Source: CAD feature listing. Evaluate the final solid. Frame: model axes, mm. Face numbers are marked on the shaded views. A direction names the side the tool comes from. Give positions to 0.01 mm unless a question says otherwise; leave off trailing zeros. Write each loop counter-clockwise with the first axis right and the second up, starting at its lowest first coordinate (ties: lowest second). Pieces come first, ordered by that corner, then holes. Notation, with made-up numbers: (17, 71.25) -> (41, 71.25) arc R12 ccw to (41, 85.25) -> close; hole circle Ø10 at (86.25, 24.25). An arc over 180 degrees is marked (long way). Write item = value, one per line.
Autodesk Inventor part; units mm, degrees
ref_plane "YZ Plane" through (0, 0, 0) normal (1, 0, 0) x (0, 1, 0)
ref_plane "XZ Plane" through (0, 0, 0) normal (0, 1, 0) x (-1, 0, 0)
ref_plane "XY Plane" through (0, 0, 0) normal (0, 0, 1) x (1, 0, 0)
sketch "Sketch1" plane through (0, 0, 0) normal (1, 0, 0) x (0, 1, 0)
  circle A0 centre (0, 0) radius 1.45
  circle A1 centre (0, -31) radius 1.45
  circle A2 centre (-31, -31) radius 1.45
  circle A3 centre (-31, 0) radius 1.45
  line L0 (0, 4.5) -> (-31, 4.5)
  line L1 (-31, 4.5) -> (-35.5, 4.5)
  line L2 (-35.5, 4.5) -> (-35.5, -35.5)
  line L3 (-35.5, -35.5) -> (4.5, -35.5)
  line L4 (4.5, -35.5) -> (4.5, 4.5)
  line L5 (4.5, 4.5) -> (0, 4.5)
  arc A4 (-4.5, 0) -> (0, -4.5) centre (0, 0) ccw
  arc A5 (-26.5, -31) -> (-31, -26.5) centre (-31, -31) ccw
  line L6 (-26.5, 0) -> (-26.5, 1.5)
  line L7 (-31, -4.5) -> (-32.5, -4.5)
  line L8 (-31, -26.5) -> (-32.5, -26.5)
  line L9 (-26.5, -31) -> (-26.5, -32.5)
  line L10 (-4.5, -31) -> (-4.5, -32.5)
  line L11 (0, -26.5) -> (1.5, -26.5)
  line L12 (0, -4.5) -> (1.5, -4.5)
  line L13 (-4.5, 0) -> (-4.5, 1.5)
  arc A6 (0, -26.5) -> (-4.5, -31) centre (0, -31) ccw
  arc A7 (-31, -4.5) -> (-26.5, 0) centre (-31, 0) ccw
  line L14 (-26.5, 1.5) -> (-4.5, 1.5)
  line L15 (1.5, -4.5) -> (1.5, -26.5)
  line L16 (-4.5, -32.5) -> (-26.5, -32.5)
  line L17 (-32.5, -26.5) -> (-32.5, -4.5)
extrude "Extrusion1" add sketch "Sketch1" along normal blind 18.2
fillet "Fillet1" radius 2 4 edges at (9.1, 4.5, 4.5) (9.1, 4.5, -35.5) (9.1, -35.5, 4.5) (9.1, -35.5, -35.5)
sketch "Sketch2" plane through (18.2, 0, 0) normal (1, 0, 0) x (0, 0, -1)
  circle A0 centre (0, 0) radius 1.45
  circle A1 centre (0, 0) radius 1.525
  circle A2 centre (31, 0) radius 1.45
  circle A3 centre (31, 0) radius 1.525
  circle A4 centre (31, -31) radius 1.45
  circle A5 centre (31, -31) radius 1.525
  circle A6 centre (0, -31) radius 1.45
  circle A7 centre (0, -31) radius 1.525
  dimension "d20" = 3.05
  dimension "d21" = 3.05
  dimension "d22" = 3.05
  dimension "d23" = 3.05
extrude "Extrusion2" cut sketch "Sketch2" against normal up to surface (18.2 mm away)
properties part number "encoder_cover"
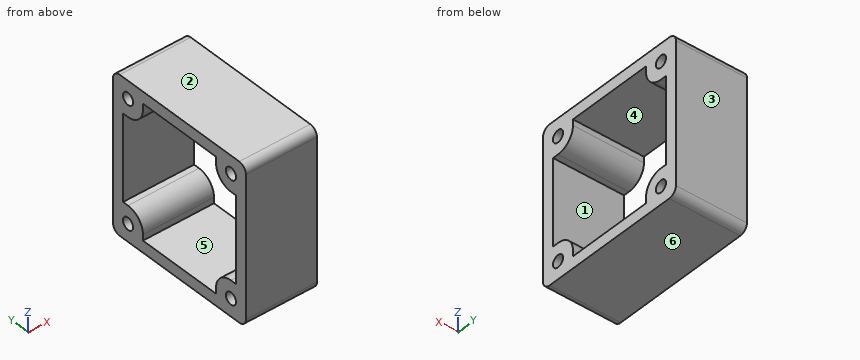
(1) Section query A-A (z = -24). Return loops of the section in (x, y), plus the area to 3 significant figures.
Values follow:
outline = (0, -35.5) -> (18.2, -35.5) -> (18.2, -32.5) -> (0, -32.5) -> close; (0, 1.5) -> (18.2, 1.5) -> (18.2, 4.5) -> (0, 4.5) -> close
area = 109 mm2
(2) Pull-direction query (Y, two-part tool) for the marked faces 3, 4, 5 and 6; classes: pulls with the +Y half, pulls with the -Y half, needs draft (parallel to the pull), parting line crosses it, or undercut.
Values follow:
face_3 = pulls with the +Y half
face_4 = undercut
face_5 = undercut
face_6 = needs draft
(3) Section query C-C (z = -32). Return loops of the section in (x, y).
Values follow:
outline = (0, -35.5) -> (18.2, -35.5) -> (18.2, -32.15) -> (0, -32.15) -> close; (0, -29.85) -> (18.2, -29.85) -> (18.2, -26.5) -> (0, -26.5) -> close; (0, -4.5) -> (18.2, -4.5) -> (18.2, -1.15) -> (0, -1.15) -> close; (0, 1.15) -> (18.2, 1.15) -> (18.2, 4.5) -> (0, 4.5) -> close
(4) Section query D-D (z = -28). Return loops of the section in (x, y), plus the area to 3 significant figures.
Values follow:
outline = (0, -35.5) -> (18.2, -35.5) -> (18.2, -27.65) -> (0, -27.65) -> close; (0, -3.35) -> (18.2, -3.35) -> (18.2, 4.5) -> (0, 4.5) -> close
area = 286 mm2
(5) Access query for the marked faces 1 and 2. Directions: +Z, -Z, +X, -X, +Y, -Y. A direction counts if a zero-diameter tool reaches every point of the face in a straight line with its end or side. Return the directions, or none.
Values follow:
face_1 = +X, -X
face_2 = +Z, +X, -X, +Y, -Y
(6) First-contact query: pin 1 (2.5 mm diameter, centred on y = 0, z = -31, fed in from -X). Flat tip, straight axial feed; report the tip coordinate or a pass-through.
Values follow:
pin_1 = through
(7) Section query B-B (x = 16.5). Return loops of the section in (y, z) (3 decimals).
Values follow:
outline = (-35.5, -33.5) arc R2 ccw to (-33.5, -35.5) -> (2.5, -35.5) arc R2 ccw to (4.5, -33.5) -> (4.5, 2.5) arc R2 ccw to (2.5, 4.5) -> (-33.5, 4.5) arc R2 ccw to (-35.5, 2.5) -> close; hole circle Ø3.05 at (-31, -31); hole circle Ø3.05 at (-31, 0); hole (-32.5, -26.5) -> (-31, -26.5) arc R4.5 cw to (-26.5, -31) -> (-26.5, -32.5) -> (-4.5, -32.5) -> (-4.5, -31) arc R4.5 cw to (0, -26.5) -> (1.5, -26.5) -> (1.5, -4.5) -> (0, -4.5) arc R4.5 cw to (-4.5, 0) -> (-4.5, 1.5) -> (-26.5, 1.5) -> (-26.5, 0) arc R4.5 cw to (-31, -4.5) -> (-32.5, -4.5) -> close; hole circle Ø3.05 at (0, -31); hole circle Ø3.05 at (0, 0)
(8) Material intervals for line 1 (Y direction, x = 5.5, z = -31) (3 decimals); line 2 (Z direction, x = 9.5, y = -23), sorted ascending.
Values follow:
line_1 = -35.5 to -32.525, -29.475 to -26.5, -4.5 to -1.525, 1.525 to 4.5
line_2 = -35.5 to -32.5, 1.5 to 4.5
